For this review, take the finished solid that the model builds, in its own axes (mm). Face numbers are marked on the shaded views. A direction names the side the tool comes from. Coordinates: 2 decimals unless noted, no trailing zeros. Order: outer loops, then holes, each group sorted by start corner. A loop starts at its lowest first (then second) coordinate and runs counter-clockwise, first axis right, second up. Notation, with made-up numbers: (60.5, -14.75) -> (77.5, -14.75) arc R31 ccw to (77.5, 15.25) -> close; hole circle Ø8 at (83, 54.25). An arc over 180 degrees is marked (long way). Answer as a JSON object with one key per item and string values. Group by question number.
1) Wall thickness on L1, parallel to Y at x = -51.5, z = -0.2; L2, parallel to X at y = -7, z = -0.7; L3, parallel to Y at x = -46.5, z = -0.15: over which ranges is each line inside the solid? List them lowest first.
2) Add section C-C, the plane z = -0.45. Write out the cut boundary in (x, y), then the cut area to 3 significant figures.
3) Machinability: for the marked faces 1 and 2, which of the approach directions +Z, -Z, +X, -X, +Y, -Y give a long, thin tool a straight path to every point of the face, cutting with its end or side? Answer none if there is none.
4) Add section B-B, the plane y = 8.5. Write out the cut boundary in (x, z).
5) For pin 1 (2.5 mm diameter, centred on x = -55.99, y = 4.31, fed in from +Z), flat-tipped, find the tip position at first contact; note if it passes through.
6) Add section A-A, the plane x = -53. Write out the cut boundary in (y, z).
from build123d import *

# Parameters (mm, degrees)
SKETCH1_W           = 40
SKETCH1_H           = 60
BOSS_EXTRUDE4_DEPTH = 3
SKETCH5_W           = 15
SKETCH5_H           = 25
CUT_EXTRUDE2_DEPTH  = 1
SKETCH7_R           = 1
CUT_EXTRUDE3_DEPTH  = 2
SKETCH8_R           = 1
CUT_EXTRUDE4_DEPTH  = 2
FILLET1_R           = 5
SKETCH12_R          = 1
CUT_EXTRUDE6_DEPTH  = 12


with BuildPart() as part:
    # Sketch1 → Boss-Extrude4 (new body)
    with BuildSketch(Plane.XY):
        with Locations((-45.9850693, -3.193565597)):
            Rectangle(SKETCH1_W, SKETCH1_H)
    extrude(amount=-BOSS_EXTRUDE4_DEPTH)

    # Sketch5 → Cut-Extrude2 (cut)
    with BuildSketch(Plane.XY):
        with Locations((-58.4850693, -3.193565597)):
            Rectangle(SKETCH5_W, SKETCH5_H)
    extrude(amount=-CUT_EXTRUDE2_DEPTH, mode=Mode.SUBTRACT)

    # Sketch7 → Cut-Extrude3 (cut)
    with BuildSketch(Plane.XY.offset(-1)):
        with Locations((-55.9850693, 4.306434403)):
            Circle(SKETCH7_R)
    extrude(amount=-CUT_EXTRUDE3_DEPTH, mode=Mode.SUBTRACT)

    # Sketch8 → Cut-Extrude4 (cut)
    with BuildSketch(Plane.XY.offset(-1)):
        with Locations((-55.9850693, -10.693565597)):
            Circle(SKETCH8_R)
    extrude(amount=-CUT_EXTRUDE4_DEPTH, mode=Mode.SUBTRACT)

    # Fillet1
    fillet1_edges = [part.edges().sort_by_distance(p)[0] for p in [
        (-65.9850693, 26.806434403, -1.5),
        (-65.9850693, -33.193565597, -1.5),
        (-25.9850693, -33.193565597, -1.5),
        (-25.9850693, 26.806434403, -1.5),
    ]]
    fillet(fillet1_edges, radius=FILLET1_R)

    # Sketch12 → Cut-Extrude6 (cut)
    with BuildSketch(Plane(origin=(0, 0, -3), x_dir=(-1, 0, 0), z_dir=(0, 0, -1))):
        with Locations((45.9850693, -3.193565597)):
            Circle(SKETCH12_R)
    extrude(amount=-CUT_EXTRUDE6_DEPTH, mode=Mode.SUBTRACT)


solid = part.part
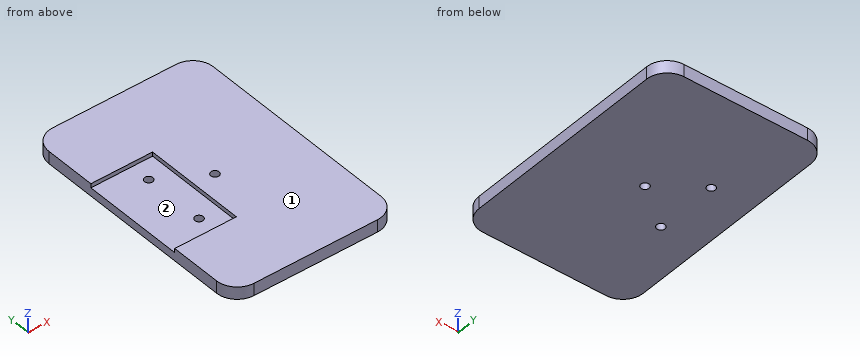
Output values:
{
 "1": {"L1": "y = -33.19 to -15.69, 9.31 to 26.81", "L2": "x = -50.99 to -25.99", "L3": "y = -33.19 to -4.05, -2.34 to 26.81"},
 "2": {"outline": "(-65.99, -28.19) arc R5 ccw to (-60.99, -33.19) -> (-30.99, -33.19) arc R5 ccw to (-25.99, -28.19) -> (-25.99, 21.81) arc R5 ccw to (-30.99, 26.81) -> (-60.99, 26.81) arc R5 ccw to (-65.99, 21.81) -> (-65.99, 9.31) -> (-50.99, 9.31) -> (-50.99, -15.69) -> (-65.99, -15.69) -> close; hole circle Ø2 at (-45.99, -3.19)", "area": "2,000 mm²"},
 "3": {"face 1": "+Z, +X, -X, +Y, -Y", "face 2": "+Z, -X"},
 "4": {"outline": "(-65.99, -3) -> (-25.99, -3) -> (-25.99, 0) -> (-50.99, 0) -> (-50.99, -1) -> (-65.99, -1) -> close"},
 "5": {"pin 1": "stops at z = -1"},
 "6": {"outline": "(-33.19, -3) -> (26.81, -3) -> (26.81, 0) -> (9.31, 0) -> (9.31, -1) -> (-15.69, -1) -> (-15.69, 0) -> (-33.19, 0) -> close"}
}
